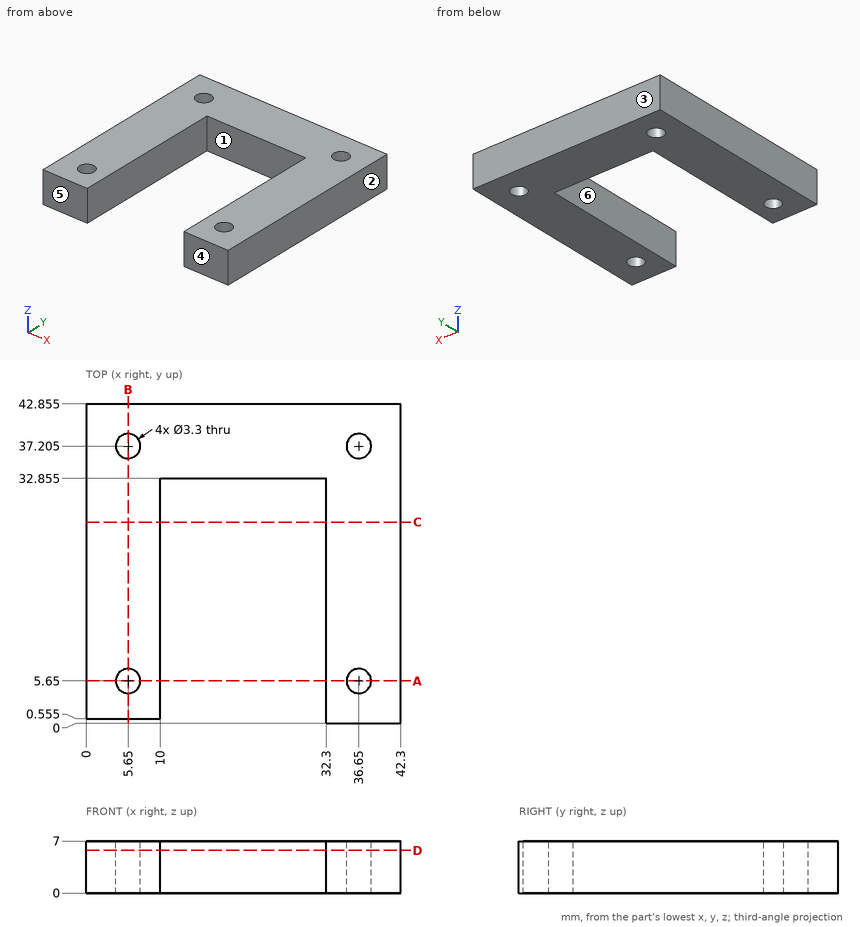
The figure shows three views and two pictorial views of one solid part (mm, origin at its lowest corner). Answer the questions. A direction names the side the tool comes from. Round coordinates to 2 decimals unless told otherwise and drop trailing zeros. Write each loop counter-clockwise with the first axis right and the second up, starting at its lowest first coordinate (ties: lowest second). Pieces come first, ordered by that corner, then holes. Notation, with made-up numbers: (89.5, 59) - (111.5, 59) arc R35 ccw to (111.5, 94) - close; hole circle Ø5 at (16.25, 45.25). An arc over 180 degrees is marked (long way). Answer in a Markdown table with one row per item. Add a question column.
1. The mould has two halves that part along X. Classify the marked faces 1, 2 and 3: +X half, -X half, draft (parallel to the pull), parting line (faces both ways), or undercut.
2. Find the intervals of material crossed by line 1 along X through (y, z) = (5.65, 4.25); line 2 along Y through (x, z) = (5.65, 5.25) (1 decimal); line 3 along Y through (x, z) = (36.65, 4.25) (1 decimal), in increasing order. Write a range as from..to.
3. A cutting plane is placed at D-D, the plane z = 5.75. Count the separate pieces of the cut face and the enclosed holes in it, and give its area (3 significant figures).
4. For the marked faces 4, 5 and 6, determine the directions among +Z, -Z, +X, -X, +Y, -Y from which every point of the face is accessible in a straight line to the end or side of a thin tool.
5. A cutting plane is placed at C-C, the plane y = 27. Determine the outline of the cut face in (x, z), and give its area (3 significant figures).
6. A cutting plane is placed at A-A, the plane y = 5.65. Determine the outline of the cut face in (x, z).
7. A cutting plane is placed at B-B, the plane x = 5.65. Determine the outline of the cut face in (y, z) (1 decimal), and give its area (3 significant figures).
8. Given pin 1 (2 mm diameter, centred on x = 36.65, y = 5.65, fed in from +Z); pin 2 (3 mm diameter, centred on x = 7.5, z = 2, fed in from -Y) (1 decimal); pin 3 (3.5 mm diameter, centred on x = 18, z = 4.5, fed in from -Y) (1 decimal), each flat-ended and moving along its own axis, determine where each tip first touches the part or whether it passes through.
Worked out:
| question | item | result |
|---|---|---|
| 1 | face 1 | undercut |
| 1 | face 2 | +X half |
| 1 | face 3 | draft |
| 2 | line 1 | 0..4, 7.3..10, 32.3..35, 38.3..42.3 |
| 2 | line 2 | 0.6..4, 7.3..35.6, 38.9..42.9 |
| 2 | line 3 | 0..4, 7.3..35.6, 38.9..42.9 |
| 3 | separate pieces | 1 |
| 3 | enclosed holes | 4 |
| 3 | area | 1,040 mm^2 |
| 4 | face 4 | +Z, -Z, +X, -X, -Y |
| 4 | face 5 | +Z, -Z, -X, -Y |
| 4 | face 6 | +Z, -Z, -Y |
| 5 | outline | (0, 0) - (10, 0) - (10, 7) - (0, 7) - close; (32.3, 0) - (42.3, 0) - (42.3, 7) - (32.3, 7) - close |
| 5 | area | 140 mm^2 |
| 6 | outline | (0, 0) - (4, 0) - (4, 7) - (0, 7) - close; (7.3, 0) - (10, 0) - (10, 7) - (7.3, 7) - close; (32.3, 0) - (35, 0) - (35, 7) - (32.3, 7) - close; (38.3, 0) - (42.3, 0) - (42.3, 7) - (38.3, 7) - close |
| 7 | outline | (0.6, 0) - (4, 0) - (4, 7) - (0.6, 7) - close; (7.3, 0) - (35.6, 0) - (35.6, 7) - (7.3, 7) - close; (38.9, 0) - (42.9, 0) - (42.9, 7) - (38.9, 7) - close |
| 7 | area | 250 mm^2 |
| 8 | pin 1 | through |
| 8 | pin 2 | y = 0.6 |
| 8 | pin 3 | y = 32.9 |
